Job drawing, mm, ordinate dimensions from the low corner. One solid piece. A direction names the side the tool comes from. Give positions to 0.01 mm unless a question says otherwise; leave off trailing zeros. Order: outer loops, then holes, each group sorted by start corner. A loop starts at its lowest first (then second) coordinate and runs counter-clockwise, first axis right, second up. Notation, with made-up numbers: M 71.25,64.25 L 88.25,64.25 A22 ccw 88.25,83.25 Z; hole C 3.5,30 d5. An arc over 180 degrees is marked long. Put each result on its own line as item: value. Start each with the question number.
1) Drill centre lines: line 1 (X direction, y = 45, z = 76); line 2 (X direction, y = 27, z = 52); line 3 (Y direction, x = 41.5, z = 96). Where is each one in solid material? Low to high. Write a range as [from, to].
2) Cut at A-A (y = 20). Give the number of separate pieces and of enclosed holes in the cut face, and give its area (3 significant figures).
3) Cut at B-B (x = 34). Write the cut outline in (y, z), and give its area (3 significant figures).
4) Two-plate mould, pull along Y, no slides. Class the marked faces 4, 5, 6 and 7: released by +Y, released by -Y, zero draft, split by the parting line, or undercut.
5) Pin check, flat tips, straight feed: pin 1 (3 mm diameter, centred on y = 13.5, z = 41.5, fed in from +X); pin 2 (1.5 mm diameter, centred on x = 31.5, y = 43.5, fed in from +Z). Stop position of each tip, or through.
6) Tool access for the marked faces 1, 2 and 3: list every direction of +Z, -Z, +X, -X, +Y, -Y with a clear straight run to the whole face (end or side of a thin tool).
7) Cut at C-C (z = 66). Write the cut outline in (x, y) (1 decimal).
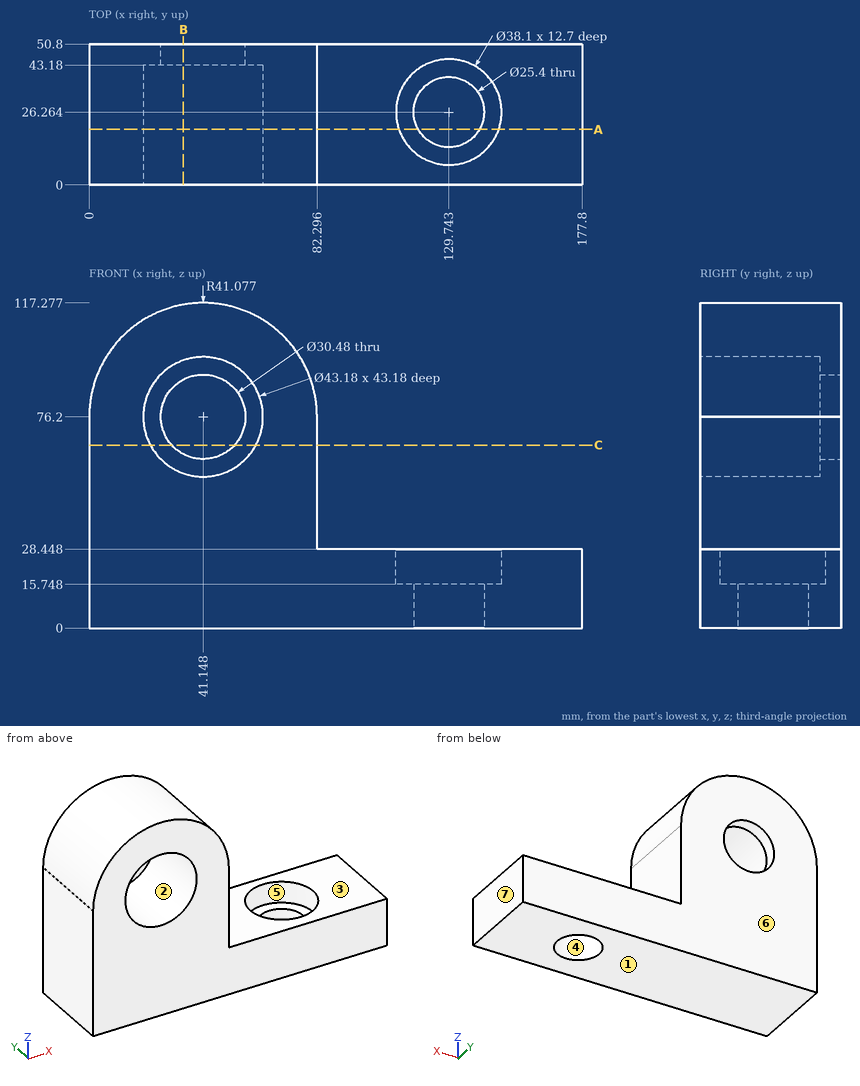
Solution:
1. line 1: [0, 25.91], [56.39, 82.3]
1. line 2: [0, 82.3]
1. line 3: [43.18, 50.8]
2. separate pieces: 2
2. enclosed holes: 1
2. area: 9,370 mm²
3. outline: M 0,0 L 50.8,0 L 50.8,62.74 L 43.18,62.74 L 43.18,55.83 L 0,55.83 Z; M 0,96.57 L 43.18,96.57 L 43.18,89.66 L 50.8,89.66 L 50.8,116.65 L 0,116.65 Z
3. area: 3,960 mm²
4. face 4: undercut
4. face 5: undercut
4. face 6: released by +Y
4. face 7: zero draft
5. pin 1: x = 82.3
5. pin 2: z = 116.3
6. face 1: -Z, +X, -X, +Y, -Y
6. face 2: -Y
6. face 3: +Z, +X, +Y, -Y
7. outline: M 0,0 L 22.1,0 L 22.1,43.2 L 29.8,43.2 L 29.8,50.8 L 0,50.8 Z; M 52.5,43.2 L 60.2,43.2 L 60.2,0 L 82.3,0 L 82.3,50.8 L 52.5,50.8 Z
